Input: part model. Units: mm. Frame: model coordinates. A direction names the side the tool comes from. Give positions to 0.01 mm unless a question says otherwise; leave off trailing zeros. Loops run counter-clockwise (first coordinate to the right, second up) from the corner with the lowest first, then second, coordinate; pieces in that order, holes last. Notation, with made-up numbers: (22, 84) - (35, 84) arc R17 ccw to (35, 113) - close; hole circle Ø1 at (-8, 42). An arc over 180 degrees is marked (long way). One line per item, written item: value.
from build123d import *

# Parameters (mm, degrees)
SKETCH1_W                      = 125
SKETCH1_H                      = 30
BOSS_EXTRUDE1_DEPTH            = 3
SKETCH2_W                      = 125
SKETCH2_H                      = 3
BOSS_EXTRUDE2_DEPTH            = 27
F_6_5_6_5_DIAMETER_HOLE1_D     = 6.5
F_6_5_6_5_DIAMETER_HOLE1_DEPTH = 10
F_6_5_6_5_DIAMETER_HOLE1_TIP   = 1.952797012
F_6_5_6_5_DIAMETER_HOLE2_D     = 6.5
F_6_5_6_5_DIAMETER_HOLE2_DEPTH = 32
F_6_5_6_5_DIAMETER_HOLE2_TIP   = 1.952797012


with BuildPart() as part:
    # Sketch1 → Boss-Extrude1 (new body)
    with BuildSketch(Plane.XY):
        Rectangle(SKETCH1_W, SKETCH1_H)
    extrude(amount=BOSS_EXTRUDE1_DEPTH)

    # Sketch2 → Boss-Extrude2 (add)
    with BuildSketch(Plane.XY.offset(3)):
        with Locations((0, -13.5)):
            Rectangle(SKETCH2_W, SKETCH2_H)
    extrude(amount=BOSS_EXTRUDE2_DEPTH)

    # Ø6.5 (6.5) Diameter Hole1
    with Locations(Plane(origin=(0, -12, 0), x_dir=(1, 0, 0), z_dir=(0, 1, 0))):
        with Locations((48.5, -15), (-50.5, -15)):
            Hole(F_6_5_6_5_DIAMETER_HOLE1_D / 2, depth=F_6_5_6_5_DIAMETER_HOLE1_DEPTH)
            with Locations((0, 0, -(F_6_5_6_5_DIAMETER_HOLE1_DEPTH + F_6_5_6_5_DIAMETER_HOLE1_TIP / 2))):  # 118° drill point
                Cone(0, F_6_5_6_5_DIAMETER_HOLE1_D / 2, F_6_5_6_5_DIAMETER_HOLE1_TIP, mode=Mode.SUBTRACT)

    # Ø6.5 (6.5) Diameter Hole2
    with Locations(Plane(origin=(0, 0, 0), x_dir=(-1, 0, 0), z_dir=(0, 0, -1))):
        with Locations((8.000002921, 7)):
            Hole(F_6_5_6_5_DIAMETER_HOLE2_D / 2, depth=F_6_5_6_5_DIAMETER_HOLE2_DEPTH)
            with Locations((0, 0, -(F_6_5_6_5_DIAMETER_HOLE2_DEPTH + F_6_5_6_5_DIAMETER_HOLE2_TIP / 2))):  # 118° drill point
                Cone(0, F_6_5_6_5_DIAMETER_HOLE2_D / 2, F_6_5_6_5_DIAMETER_HOLE2_TIP, mode=Mode.SUBTRACT)


solid = part.part
Item 1: Material intervals for L1, parallel to X at y = -13.75, z = 15; L2, parallel to Z at x = 48.5, y = -13.2; L3, parallel to Y at x = -26.5, z = 8.5, sorted ascending.
Verdict:
L1: x = -62.5 to -53.75, -47.25 to 45.25, 51.75 to 62.5
L2: z = 0 to 11.75, 18.25 to 30
L3: y = -15 to -12
Item 2: Access query for faces 1 (the face through (-1, 15, 1)), 2 (the face through (-1, 2, 3)). Directions: +Z, -Z, +X, -X, +Y, -Y. A direction counts if a zero-diameter tool reaches every point of the face in a straight line with its end or side. Return the directions, or none.
Verdict:
face 1: +Z, -Z, +X, -X, +Y
face 2: +Z, +X, -X, +Y
Item 3: Section D-D, the plane x = 50.5. Output: boundary loops of the cut face in (y, z).
Verdict:
outline: (-15, 0) - (15, 0) - (15, 3) - (-12, 3) - (-12, 12.44) - (-15, 12.44) - close; (-15, 17.56) - (-12, 17.56) - (-12, 30) - (-15, 30) - close
Item 4: Section C-C, the plane z = 15. Output: boundary loops of the cut face in (x, y).
Verdict:
outline: (-62.5, -15) - (-53.75, -15) - (-53.75, -12) - (-62.5, -12) - close; (-47.25, -15) - (45.25, -15) - (45.25, -12) - (-47.25, -12) - close; (51.75, -15) - (62.5, -15) - (62.5, -12) - (51.75, -12) - close
Item 5: Section A-A, the plane y = 8.25. Output: boundary loops of the cut face in (x, z), and give its area (3 significant figures).
Verdict:
outline: (-62.5, 0) - (-11, 0) - (-11, 3) - (-62.5, 3) - close; (-5, 0) - (62.5, 0) - (62.5, 3) - (-5, 3) - close
area: 357 mm^2
Item 6: Draft query along X for faces 3 (the face through (62.5, -12.3, 8.3)), 4 (the face through (-1, -12, 16)), 5 (the face through (45.4, -13.52, 14.02)). Return one class per face: pulls with the +X half, pulls with the -X half, needs draft (parallel to the pull), parting line crosses it, or undercut.
Verdict:
face 3: pulls with the +X half
face 4: needs draft
face 5: undercut
Item 7: Pin query (flat end, axial travel): P1, Ø4, axis at x = 10.5, z = 13.5, coming from the +Y side; P2, Ø4, axis at x = -8, y = 7, coming from the +Z side. Return the tip coordinate at first contact, or that it passes through.
Verdict:
P1: stops at y = -12
P2: passes through
Item 8: Section B-B, the plane x = -50.5. Output: boundary loops of the cut face in (y, z), and give its area (4 significant figures).
Verdict:
outline: (-15, 0) - (15, 0) - (15, 3) - (-12, 3) - (-12, 11.75) - (-15, 11.75) - close; (-15, 18.25) - (-12, 18.25) - (-12, 30) - (-15, 30) - close
area: 151.5 mm^2
